Autodesk Fusion 360 part; units mm, degrees
sketch "Sketch1" plane through (0, 0, 0) normal (0, 0, 1) x (1, 0, 0)
  line L0 (0, 0) -> (90, 0)
  line L1 (90, 0) -> (90, 60)
  line L2 (90, 60) -> (0, 60)
  line L3 (0, 60) -> (0, 0)
  circle A0 centre (45, 19) radius 3
  circle A1 centre (13, 19) radius 4
  circle A2 centre (77, 19) radius 4
  circle A3 centre (45, 44) radius 7.5
  line L4 (22.6906, 1) -> (27.3094, 1)
  line L5 (27.3094, 1) -> (29.6188, 5)
  line L6 (29.6188, 5) -> (27.3094, 9)
  line L7 (27.3094, 9) -> (22.6906, 9)
  line L8 (22.6906, 9) -> (20.3812, 5)
  line L9 (20.3812, 5) -> (22.6906, 1)
  line L10 (67.3524, 8.9748) -> (62.7339, 9.0247)
  line L11 (62.7339, 9.0247) -> (60.3815, 5.0499)
  line L12 (60.3815, 5.0499) -> (62.6476, 1.0252)
  line L13 (62.6476, 1.0252) -> (67.2661, 0.9753)
  line L14 (67.2661, 0.9753) -> (69.6185, 4.9501)
  line L15 (69.6185, 4.9501) -> (67.3524, 8.9748)
  circle A4 centre (25, 5) radius 2.5
  circle A5 centre (65, 5) radius 2.5
  circle A6 centre (45, 44) radius 12
  circle A7 centre (77, 19) radius 7
  circle A8 centre (45, 19) radius 6
  circle A9 centre (13, 19) radius 7
  point P0 (25, 5)
  point P1 (65, 5)
  dimension "d4" = 90
  dimension "d5" = 60
  dimension "d6" = 45
  dimension "d7" = 32
  dimension "d8" = 32
  dimension "d9" = 19
  dimension "d10" = 19
  dimension "d11" = 19
  dimension "d12" = 25
  dimension "d16" = 8
  dimension "d17" = 25
  dimension "d19" = 5
  dimension "d20" = 8
  dimension "d21" = 40
  dimension "d22" = 5
extrude "Extrude1" add sketch "Sketch1" along normal blind 10 contours L0 L1 L2 L3 | L4 L5 L6 L7 L8 L9 | L10 L11 L12 L13 L14 L15 | A6 | A7 | A8 | A9
extrude "Extrude2" cut sketch "Sketch1" along normal blind 10 and the other way blind -6 contours L4 L5 L6 L7 L8 L9 | L10 L11 L12 L13 L14 L15
extrude "Extrude3" add sketch "Sketch1" along normal blind 16 contours A6 | A7 | A8 | A9
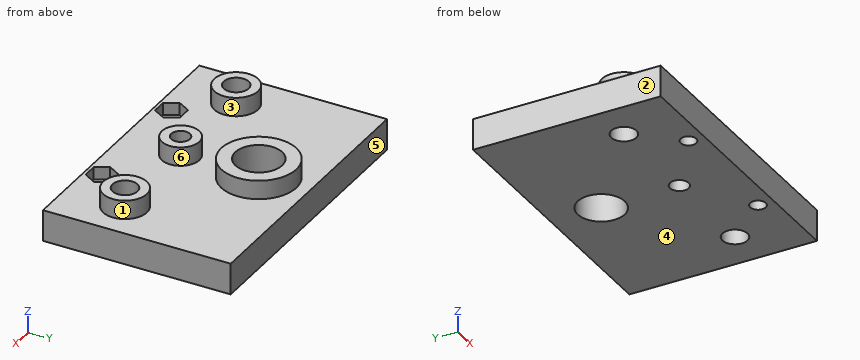
Input: part model. Units: mm. Frame: model coordinates. Face numbers are marked on the shaded views. A direction names the side the tool comes from. Round coordinates to 2 decimals unless told otherwise and drop trailing zeros. Order: outer loops, then holes, each group sorted by start corner. A loop starts at its lowest first (then second) coordinate and runs counter-clockwise, first axis right, second up. Notation, with made-up numbers: (16.5, -20) - (70.5, -20) arc R15 cw to (70.5, 0) - close; hole circle Ø3 at (54, 51.25). An arc over 180 degrees is marked (long way). Answer as a JSON object with one key per item and string values. Group by question number.
(1) Cut plane D-D (x = 77). Return loops of the section in (y, z), then the cut area to 3 significant figures.
(2) Cut plane C-C (z = 4.5). Return loops of the section in (x, y), then the cut area to 3 significant figures.
(3) Material intervals for probe 1 along Y at (x, z) = (45, 9); probe 2 along Y at (x, z) = (25, 2.35); probe 3 along Y at (x, z) = (45, 12), sorted ascending. Write a range as from..to.
(4) Cut plane A-A (z = 11.75). Return loops of the section in (x, y).
(5) Reachability of the marked faces 1 and 2 from +Z, -Z, +X, -X, +Y, -Y: full face, straight path, thin tool, end or side. Return the list, or none.
(6) Pin query (flat end, axial travel): P1, Ø2, axis at x = 78.5, z = 11.5, coming from the -Y side; P2, Ø1.5, axis at x = 14, y = 21, coming from the -Z side; P3, Ø3, axis at x = 20, z = 13, coming from the -Y side; P4, Ø4, axis at x = 67, y = 5, coming from the +Z side. Return the tip coordinate at first contact, or that it passes through.
(7) Cut plane B-B (y = 44). Return loops of the section in (x, z), then the cut area to 3 significant figures.
(8) Draft query along Y for the marked faces 3, 4, 5 and 6. Return one class per face: released by +Y, released by -Y, zero draft, split by the parting line, or undercut.
Here are the results:
{
 "1": {"outline": "(0, 0) - (15, 0) - (15, 16) - (12, 16) - (12, 10) - (0, 10) - close; (23, 0) - (60, 0) - (60, 10) - (26, 10) - (26, 16) - (23, 16) - close", "area": "556 mm^2"},
 "2": {"outline": "(0, 0) - (90, 0) - (90, 60) - (0, 60) - close; hole circle Ø8 at (13, 19); hole circle Ø5 at (25, 5); hole circle Ø15 at (45, 44); hole circle Ø6 at (45, 19); hole circle Ø5 at (65, 5); hole circle Ø8 at (77, 19)", "area": "5,060 mm^2"},
 "3": {"probe 1": "y = 0..16, 22..36.5, 51.5..60", "probe 2": "y = 0..2.5, 7.5..60", "probe 3": "y = 13..16, 22..25, 32..36.5, 51.5..56"},
 "4": {"outline": "circle Ø14 at (13, 19); circle Ø24 at (45, 44); circle Ø12 at (45, 19); circle Ø14 at (77, 19); hole circle Ø8 at (13, 19); hole circle Ø15 at (45, 44); hole circle Ø6 at (45, 19); hole circle Ø8 at (77, 19)"},
 "5": {"face 1": "+Z", "face 2": "+Z, -Z, -X, +Y, -Y"},
 "6": {"P1": "stops at y = 12.02", "P2": "passes through", "P3": "stops at y = 14.67", "P4": "stops at z = 6"},
 "7": {"outline": "(0, 0) - (37.5, 0) - (37.5, 16) - (33, 16) - (33, 10) - (0, 10) - close; (52.5, 0) - (90, 0) - (90, 10) - (57, 10) - (57, 16) - (52.5, 16) - close", "area": "804 mm^2"},
 "8": {"face 3": "split by the parting line", "face 4": "zero draft", "face 5": "released by +Y", "face 6": "undercut"}
}
